Drawing for the job (mm, zero at the part's lowest x, y, z). Coordinates: 2 decimals unless noted, no trailing zeros. Order: outer loops, then holes, each group sorted by start corner. A loop starts at its lowest first (then second) coordinate and runs counter-clockwise, first axis right, second up.
1) Wall check: L1, parallel to Y at x = 154, z = 95; L2, parallel to X at y = 8.5, z = 129. Give the ranges that are in metal, low to high.
2) Pin check, flat tips, straight feed: pin 1 Ø2.5 at (y, z) = (59.5, 110.5) entering from +X; pin 2 Ø6 at (y, z) = (71.5, 110.5) entering from -X; pin 3 Ø4.5 at (x, y) = (86, 56.5) entering from -Z (3 decimals). Stop position of each tip, or through.
3) Cut at B-B (z = 86.5). List the corners of the cut face in (x, y), and give its area (3 significant figures).
4) Cut at A-A (y = 107). List the corners of the cut face in (x, z) (3 decimals).
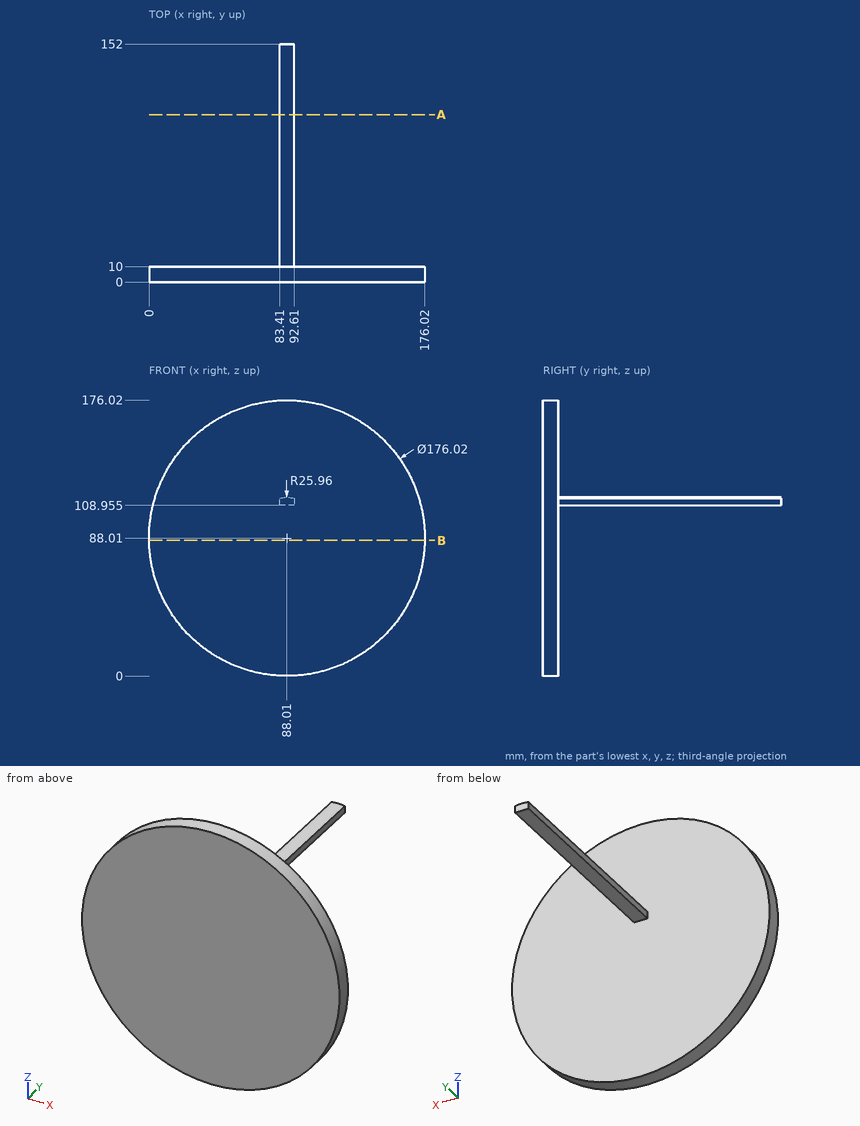
Geometry check:
1. L1: y = 0 to 10
1. L2: x = 10.13 to 165.89
2. pin 1: stops at x = 92.61
2. pin 2: stops at x = 83.41
2. pin 3: stops at z = 108.955
3. outline: (0.01, 0) - (176.01, 0) - (176.01, 10) - (0.01, 10) - close
3. area: 1,760 mm2
4. outline: (83.41, 108.955) - (92.61, 108.955) - (92.61, 113.559) arc R25.96 ccw to (83.41, 113.559) - close
